The listing builds one solid part. Answer for the finished solid, in the listing's coordinates (mm). Coordinates: 2 decimals unless noted, no trailing zeros. Write each loop counter-clockwise with the first axis right and the second up, starting at its lowest first coordinate (ties: lowest second). Pieces come first, ordered by that corner, then holes.
from build123d import *
from OCP.BRepFilletAPI import BRepFilletAPI_MakeChamfer

# Parameters (mm, degrees)
BOSS_EXTRU_1_DEPTH      = 12
BOSS_EXTRU_1_TAPER      = 2
CHANFREIN2_SIZE         = 0.6
CHANFREIN2_SIZE2        = 0.353753521
ENL_V_MAT_EXTRU_1_DEPTH = 10
ESQUISSE4_R             = 0.2
ENL_V_MAT_EXTRU_4_DEPTH = 10
CHANFREIN3_SIZE         = 0.2


with BuildPart() as part:
    # Esquisse1 → Boss.-Extru.1 (new body)
    with BuildSketch(Plane.XY):
        with BuildLine():
            ThreePointArc((4.472222222, -0.499227799), (4, 0), (4.472222222, 0.499227799))
            ThreePointArc((4.472222222, 0.499227799), (4.279754323, 1.390576475), (3.911542518, 2.224822494))
            ThreePointArc((3.911542518, 2.224822494), (3.236067977, 2.351141009), (3.324665043, 3.03259004))
            ThreePointArc((3.324665043, 3.03259004), (2.645033635, 3.640576475), (1.85678652, 4.099066213))
            ThreePointArc((1.85678652, 4.099066213), (1.236067977, 3.804226065), (0.907198818, 4.407605961))
            ThreePointArc((0.907198818, 4.407605961), (0, 4.5), (-0.907198818, 4.407605961))
            ThreePointArc((-0.907198818, 4.407605961), (-1.236067977, 3.804226065), (-1.85678652, 4.099066213))
            ThreePointArc((-1.85678652, 4.099066213), (-2.645033635, 3.640576475), (-3.324665043, 3.03259004))
            ThreePointArc((-3.324665043, 3.03259004), (-3.236067977, 2.351141009), (-3.911542518, 2.224822494))
            ThreePointArc((-3.911542518, 2.224822494), (-4.279754323, 1.390576475), (-4.472222222, 0.499227799))
            ThreePointArc((-4.472222222, 0.499227799), (-4, 0), (-4.472222222, -0.499227799))
            ThreePointArc((-4.472222222, -0.499227799), (-4.279754323, -1.390576475), (-3.911542518, -2.224822494))
            ThreePointArc((-3.911542518, -2.224822494), (-3.236067977, -2.351141009), (-3.324665043, -3.03259004))
            ThreePointArc((-3.324665043, -3.03259004), (-2.645033635, -3.640576475), (-1.85678652, -4.099066213))
            ThreePointArc((-1.85678652, -4.099066213), (-1.236067977, -3.804226065), (-0.907198818, -4.407605961))
            ThreePointArc((-0.907198818, -4.407605961), (0, -4.5), (0.907198818, -4.407605961))
            ThreePointArc((0.907198818, -4.407605961), (1.236067977, -3.804226065), (1.85678652, -4.099066213))
            ThreePointArc((1.85678652, -4.099066213), (2.645033635, -3.640576475), (3.324665043, -3.03259004))
            ThreePointArc((3.324665043, -3.03259004), (3.236067977, -2.351141009), (3.911542518, -2.224822494))
            ThreePointArc((3.911542518, -2.224822494), (4.279754323, -1.390576475), (4.472222222, -0.499227799))
        make_face()
    extrude(amount=BOSS_EXTRU_1_DEPTH, taper=BOSS_EXTRU_1_TAPER)

    # Chanfrein2: one chamfer whose edges measure the first distance from different faces: ONE call of the kernel's chamfer builder (chamfer() names one face for all edges)
    chanfrein2_edges_1 = [part.edges().sort_by_distance(p)[0] for p in [
        (-3.881214819, 1.26108314, 12),
    ]]
    chanfrein2_side_1 = [part.faces().sort_by_distance(p)[0] for p in [
        (-4.080484571, 1.325829807, 6),
    ]]
    chanfrein2_edges_2 = [part.edges().sort_by_distance(p)[0] for p in [
        (-2.897050026, 2.104830049, 12),
    ]]
    chanfrein2_side_2 = [part.faces().sort_by_distance(p)[0] for p in [
        (-3.066559002, 2.227985529, 6),
    ]]
    chanfrein2_edges_3 = [part.edges().sort_by_distance(p)[0] for p in [
        (-2.398722676, 3.301558523, 12),
    ]]
    chanfrein2_side_3 = [part.faces().sort_by_distance(p)[0] for p in [
        (-2.521878155, 3.471067499, 6),
    ]]
    chanfrein2_edges_4 = [part.edges().sort_by_distance(p)[0] for p in [
        (-1.106574643, 3.405686561, 12),
    ]]
    chanfrein2_side_4 = [part.faces().sort_by_distance(p)[0] for p in [
        (-1.17132131, 3.604956313, 6),
    ]]
    chanfrein2_edges_5 = [part.edges().sort_by_distance(p)[0] for p in [
        (0, 4.080950766, 12),
    ]]
    chanfrein2_side_5 = [part.faces().sort_by_distance(p)[0] for p in [
        (0, 4.290475383, 6),
    ]]
    chanfrein2_edges_6 = [part.edges().sort_by_distance(p)[0] for p in [
        (1.106574643, 3.405686561, 12),
    ]]
    chanfrein2_side_6 = [part.faces().sort_by_distance(p)[0] for p in [
        (1.17132131, 3.604956313, 6),
    ]]
    chanfrein2_edges_7 = [part.edges().sort_by_distance(p)[0] for p in [
        (2.398722676, 3.301558523, 12),
    ]]
    chanfrein2_side_7 = [part.faces().sort_by_distance(p)[0] for p in [
        (2.521878155, 3.471067499, 6),
    ]]
    chanfrein2_edges_8 = [part.edges().sort_by_distance(p)[0] for p in [
        (2.897050026, 2.104830049, 12),
    ]]
    chanfrein2_side_8 = [part.faces().sort_by_distance(p)[0] for p in [
        (3.066559002, 2.227985529, 6),
    ]]
    chanfrein2_edges_9 = [part.edges().sort_by_distance(p)[0] for p in [
        (3.881214819, 1.26108314, 12),
    ]]
    chanfrein2_side_9 = [part.faces().sort_by_distance(p)[0] for p in [
        (4.080484571, 1.325829807, 6),
    ]]
    chanfrein2_edges_10 = [part.edges().sort_by_distance(p)[0] for p in [
        (3.580950766, 0, 12),
    ]]
    chanfrein2_side_10 = [part.faces().sort_by_distance(p)[0] for p in [
        (3.790475383, 0, 6),
    ]]
    chanfrein2_edges_11 = [part.edges().sort_by_distance(p)[0] for p in [
        (3.881214819, -1.26108314, 12),
    ]]
    chanfrein2_side_11 = [part.faces().sort_by_distance(p)[0] for p in [
        (4.080484571, -1.325829807, 6),
    ]]
    chanfrein2_edges_12 = [part.edges().sort_by_distance(p)[0] for p in [
        (2.897050026, -2.104830049, 12),
    ]]
    chanfrein2_side_12 = [part.faces().sort_by_distance(p)[0] for p in [
        (3.066559002, -2.227985529, 6),
    ]]
    chanfrein2_edges_13 = [part.edges().sort_by_distance(p)[0] for p in [
        (2.398722676, -3.301558523, 12),
    ]]
    chanfrein2_side_13 = [part.faces().sort_by_distance(p)[0] for p in [
        (2.521878155, -3.471067499, 6),
    ]]
    chanfrein2_edges_14 = [part.edges().sort_by_distance(p)[0] for p in [
        (1.106574643, -3.405686561, 12),
    ]]
    chanfrein2_side_14 = [part.faces().sort_by_distance(p)[0] for p in [
        (1.17132131, -3.604956313, 6),
    ]]
    chanfrein2_edges_15 = [part.edges().sort_by_distance(p)[0] for p in [
        (0, -4.080950766, 12),
    ]]
    chanfrein2_side_15 = [part.faces().sort_by_distance(p)[0] for p in [
        (0, -4.290475383, 6),
    ]]
    chanfrein2_edges_16 = [part.edges().sort_by_distance(p)[0] for p in [
        (-1.106574643, -3.405686561, 12),
    ]]
    chanfrein2_side_16 = [part.faces().sort_by_distance(p)[0] for p in [
        (-1.17132131, -3.604956313, 6),
    ]]
    chanfrein2_edges_17 = [part.edges().sort_by_distance(p)[0] for p in [
        (-2.398722676, -3.301558523, 12),
    ]]
    chanfrein2_side_17 = [part.faces().sort_by_distance(p)[0] for p in [
        (-2.521878155, -3.471067499, 6),
    ]]
    chanfrein2_edges_18 = [part.edges().sort_by_distance(p)[0] for p in [
        (-2.897050026, -2.104830049, 12),
    ]]
    chanfrein2_side_18 = [part.faces().sort_by_distance(p)[0] for p in [
        (-3.066559002, -2.227985529, 6),
    ]]
    chanfrein2_edges_19 = [part.edges().sort_by_distance(p)[0] for p in [
        (-3.881214819, -1.26108314, 12),
    ]]
    chanfrein2_side_19 = [part.faces().sort_by_distance(p)[0] for p in [
        (-4.080484571, -1.325829807, 6),
    ]]
    chanfrein2_edges_20 = [part.edges().sort_by_distance(p)[0] for p in [
        (-3.580950766, 0, 12),
    ]]
    chanfrein2_side_20 = [part.faces().sort_by_distance(p)[0] for p in [
        (-3.790475383, 0, 6),
    ]]
    chanfrein2 = BRepFilletAPI_MakeChamfer(part.part.solid().wrapped)
    for e in chanfrein2_edges_1:
        chanfrein2.Add(CHANFREIN2_SIZE, CHANFREIN2_SIZE2, e.wrapped, chanfrein2_side_1[0].wrapped)  # the first distance lies on this face
    for e in chanfrein2_edges_2:
        chanfrein2.Add(CHANFREIN2_SIZE, CHANFREIN2_SIZE2, e.wrapped, chanfrein2_side_2[0].wrapped)  # the first distance lies on this face
    for e in chanfrein2_edges_3:
        chanfrein2.Add(CHANFREIN2_SIZE, CHANFREIN2_SIZE2, e.wrapped, chanfrein2_side_3[0].wrapped)  # the first distance lies on this face
    for e in chanfrein2_edges_4:
        chanfrein2.Add(CHANFREIN2_SIZE, CHANFREIN2_SIZE2, e.wrapped, chanfrein2_side_4[0].wrapped)  # the first distance lies on this face
    for e in chanfrein2_edges_5:
        chanfrein2.Add(CHANFREIN2_SIZE, CHANFREIN2_SIZE2, e.wrapped, chanfrein2_side_5[0].wrapped)  # the first distance lies on this face
    for e in chanfrein2_edges_6:
        chanfrein2.Add(CHANFREIN2_SIZE, CHANFREIN2_SIZE2, e.wrapped, chanfrein2_side_6[0].wrapped)  # the first distance lies on this face
    for e in chanfrein2_edges_7:
        chanfrein2.Add(CHANFREIN2_SIZE, CHANFREIN2_SIZE2, e.wrapped, chanfrein2_side_7[0].wrapped)  # the first distance lies on this face
    for e in chanfrein2_edges_8:
        chanfrein2.Add(CHANFREIN2_SIZE, CHANFREIN2_SIZE2, e.wrapped, chanfrein2_side_8[0].wrapped)  # the first distance lies on this face
    for e in chanfrein2_edges_9:
        chanfrein2.Add(CHANFREIN2_SIZE, CHANFREIN2_SIZE2, e.wrapped, chanfrein2_side_9[0].wrapped)  # the first distance lies on this face
    for e in chanfrein2_edges_10:
        chanfrein2.Add(CHANFREIN2_SIZE, CHANFREIN2_SIZE2, e.wrapped, chanfrein2_side_10[0].wrapped)  # the first distance lies on this face
    for e in chanfrein2_edges_11:
        chanfrein2.Add(CHANFREIN2_SIZE, CHANFREIN2_SIZE2, e.wrapped, chanfrein2_side_11[0].wrapped)  # the first distance lies on this face
    for e in chanfrein2_edges_12:
        chanfrein2.Add(CHANFREIN2_SIZE, CHANFREIN2_SIZE2, e.wrapped, chanfrein2_side_12[0].wrapped)  # the first distance lies on this face
    for e in chanfrein2_edges_13:
        chanfrein2.Add(CHANFREIN2_SIZE, CHANFREIN2_SIZE2, e.wrapped, chanfrein2_side_13[0].wrapped)  # the first distance lies on this face
    for e in chanfrein2_edges_14:
        chanfrein2.Add(CHANFREIN2_SIZE, CHANFREIN2_SIZE2, e.wrapped, chanfrein2_side_14[0].wrapped)  # the first distance lies on this face
    for e in chanfrein2_edges_15:
        chanfrein2.Add(CHANFREIN2_SIZE, CHANFREIN2_SIZE2, e.wrapped, chanfrein2_side_15[0].wrapped)  # the first distance lies on this face
    for e in chanfrein2_edges_16:
        chanfrein2.Add(CHANFREIN2_SIZE, CHANFREIN2_SIZE2, e.wrapped, chanfrein2_side_16[0].wrapped)  # the first distance lies on this face
    for e in chanfrein2_edges_17:
        chanfrein2.Add(CHANFREIN2_SIZE, CHANFREIN2_SIZE2, e.wrapped, chanfrein2_side_17[0].wrapped)  # the first distance lies on this face
    for e in chanfrein2_edges_18:
        chanfrein2.Add(CHANFREIN2_SIZE, CHANFREIN2_SIZE2, e.wrapped, chanfrein2_side_18[0].wrapped)  # the first distance lies on this face
    for e in chanfrein2_edges_19:
        chanfrein2.Add(CHANFREIN2_SIZE, CHANFREIN2_SIZE2, e.wrapped, chanfrein2_side_19[0].wrapped)  # the first distance lies on this face
    for e in chanfrein2_edges_20:
        chanfrein2.Add(CHANFREIN2_SIZE, CHANFREIN2_SIZE2, e.wrapped, chanfrein2_side_20[0].wrapped)  # the first distance lies on this face
    add(Compound.cast(chanfrein2.Shape()), mode=Mode.REPLACE)

    # Esquisse2 → Enlèv. mat.-Extru.1 (cut)
    with BuildSketch(Plane(origin=(0, 0, 0), x_dir=(-1, 0, 0), z_dir=(0, 0, -1))):
        with BuildLine():
            Line((-2.655183609, -1.6), (2.655183609, -1.6))
            ThreePointArc((2.655183609, -1.6), (2.986726401, -0.830340536), (3.1, 0))
            ThreePointArc((3.1, 0), (-0.830340536, 2.986726401), (-2.655183609, -1.6))
        make_face()
    extrude(amount=-ENL_V_MAT_EXTRU_1_DEPTH, mode=Mode.SUBTRACT)

    # Esquisse4 → Enlèv. mat.-Extru.4 (cut)
    with BuildSketch(Plane(origin=(0, 0, 0), x_dir=(-1, 0, 0), z_dir=(0, 0, -1))):
        with Locations((-2.655183609, -1.6)):
            Circle(ESQUISSE4_R)
        with Locations((2.598076211, -1.6)):
            Circle(ESQUISSE4_R)
    extrude(amount=-ENL_V_MAT_EXTRU_4_DEPTH, mode=Mode.SUBTRACT)

    # Chanfrein3
    chanfrein3_edges = [part.edges().sort_by_distance(p)[0] for p in [
        (0.028553699, -1.6, 0),
    ]]
    chamfer(chanfrein3_edges, length=CHANFREIN3_SIZE - 0.0001)  # a hair under: the kernel refuses the full size


solid = part.part
Q1. Given pin 1 (3.5 mm diameter, centred on x = 0, y = 0, fed in from -Z); pin 2 (1.5 mm diameter, centred on y = -0.5, z = 9, fed in from -X); pin 3 (3 mm diameter, centred on x = -2, y = -0.5, fed in from -Z); pin 4 (2.5 mm diameter, centred on x = -1, y = 1, fed in from -Z), each flat-ended and moving along its own axis, determine where each tip first touches the part or whether it passes through.
Answers below:
pin 1: stops at z = 0.05
pin 2: stops at x = -4.15
pin 3: stops at z = 0
pin 4: stops at z = 10
Q2. Determine the mould class of faces 1 (the face through (-4.084, 1.34, 5.78)), 2 (the face through (-1.188, -3.608, 5.78)), 3 (the face through (3.45, -0.01, 11.64)) for opening direction X: released by +X, released by -X, zero draft, split by the parting line, or undercut.
Answers below:
face 1: released by -X
face 2: undercut
face 3: released by +X
Q3. The part is cut by section B-B, the plane z = 7.5. Write down the section's boundary in (x, y), then the cut area to 3 significant figures.
Answers below:
outline: (-4.18, -0.69) arc R4.24 ccw to (-3.79, -1.9) arc R0.76 cw to (-2.98, -3.02) arc R4.24 ccw to (-1.95, -3.76) arc R0.76 cw to (-0.63, -4.19) arc R4.24 ccw to (0.63, -4.19) arc R0.76 cw to (1.95, -3.76) arc R4.24 ccw to (2.98, -3.02) arc R0.76 cw to (3.79, -1.9) arc R4.24 ccw to (4.18, -0.69) arc R0.76 cw to (4.18, 0.69) arc R4.24 ccw to (3.79, 1.9) arc R0.76 cw to (2.98, 3.02) arc R4.24 ccw to (1.95, 3.76) arc R0.76 cw to (0.63, 4.19) arc R4.24 ccw to (-0.63, 4.19) arc R0.76 cw to (-1.95, 3.76) arc R4.24 ccw to (-2.98, 3.02) arc R0.76 cw to (-3.79, 1.9) arc R4.24 ccw to (-4.18, 0.69) arc R0.76 cw to start; hole (-2.74, -1.46) arc R0.2 ccw (long way) to (-2.4, -1.6) - (2.46, -1.6) arc R0.2 ccw (long way) to (2.75, -1.43) arc R3.1 ccw (long way) to start
area: 26.8 mm2
Q4. The part is cut by section C-C, the plane z = 10.25. Write down the section's boundary in (x, y) (3 decimals), then the cut area to 3 significant figures.
Answers below:
outline: (-4.075, -0.745) arc R4.142 ccw to (-3.734, -1.792) arc R0.858 cw to (-2.858, -2.998) arc R4.142 ccw to (-1.968, -3.645) arc R0.858 cw to (-0.551, -4.105) arc R4.142 ccw to (0.551, -4.105) arc R0.858 cw to (1.968, -3.645) arc R4.142 ccw to (2.858, -2.998) arc R0.858 cw to (3.734, -1.792) arc R4.142 ccw to (4.075, -0.745) arc R0.858 cw to (4.075, 0.745) arc R4.142 ccw to (3.734, 1.792) arc R0.858 cw to (2.858, 2.998) arc R4.142 ccw to (1.968, 3.645) arc R0.858 cw to (0.551, 4.105) arc R4.142 ccw to (-0.551, 4.105) arc R0.858 cw to (-1.968, 3.645) arc R4.142 ccw to (-2.858, 2.998) arc R0.858 cw to (-3.734, 1.792) arc R4.142 ccw to (-4.075, 0.745) arc R0.858 cw to start
area: 48.7 mm2
Q5. Find the intervals of material crossed by probe 1 along Z at (x, y) = (2.25, 2); probe 2 along Y at (x, z) = (-0.25, 5); probe 3 along Y at (x, z) = (-0.75, 7), in increasing order.
Answers below:
probe 1: z = 10 to 12
probe 2: y = -4.32 to -1.6, 3.09 to 4.32
probe 3: y = -3.9 to -1.6, 3.01 to 3.9
Q6. The part is cut by section D-D, the plane z = 4.25. Write down the section's boundary in (x, y), then the cut area to 3 significant figures.
Answers below:
outline: (-4.31, -0.62) arc R4.35 ccw to (-3.85, -2.03) arc R0.65 cw to (-3.12, -3.03) arc R4.35 ccw to (-1.92, -3.91) arc R0.65 cw to (-0.74, -4.29) arc R4.35 ccw to (0.74, -4.29) arc R0.65 cw to (1.92, -3.91) arc R4.35 ccw to (3.12, -3.03) arc R0.65 cw to (3.85, -2.03) arc R4.35 ccw to (4.31, -0.62) arc R0.65 cw to (4.31, 0.62) arc R4.35 ccw to (3.85, 2.03) arc R0.65 cw to (3.12, 3.03) arc R4.35 ccw to (1.92, 3.91) arc R0.65 cw to (0.74, 4.29) arc R4.35 ccw to (-0.74, 4.29) arc R0.65 cw to (-1.92, 3.91) arc R4.35 ccw to (-3.12, 3.03) arc R0.65 cw to (-3.85, 2.03) arc R4.35 ccw to (-4.31, 0.62) arc R0.65 cw to start; hole (-2.74, -1.46) arc R0.2 ccw (long way) to (-2.4, -1.6) - (2.46, -1.6) arc R0.2 ccw (long way) to (2.75, -1.43) arc R3.1 ccw (long way) to start
area: 30.3 mm2
Q7. The part is cut by section A-A, the plane x = 0. Write down the section's boundary in (y, z).
Answers below:
outline: (-4.5, 0) - (-1.8, 0) - (-1.6, 0.2) - (-1.6, 10) - (3.1, 10) - (3.1, 0) - (4.5, 0) - (4.1, 11.4) - (3.73, 12) - (-3.73, 12) - (-4.1, 11.4) - close
